from build123d import *

# Parameters (mm, degrees)
PAD_DEPTH = 10


with BuildPart() as part:
    # Sketch → Pad (new body)
    with BuildSketch(Plane.XY):
        with BuildLine():
            ThreePointArc((5, 0), (0, 5), (-5, 0))
            Line((-7, 0), (-5, 0))
            Line((-7, 7.124356), (-7, 0))
            ThreePointArc((-7, 7.124356), (-3.464466, 8.588822), (-2, 12.124356))
            Line((2, 12.124356), (-2, 12.124356))
            ThreePointArc((2, 12.124356), (3.464466, 8.588822), (7, 7.124356))
            Line((7, 0), (7, 7.124356))
            Line((5, 0), (7, 0))
        make_face()
    extrude(amount=PAD_DEPTH)


solid = part.part
The listing builds one solid part. Answer for the finished solid, in the listing's coordinates (mm). Give positions to 0.01 mm unless a question says otherwise; leave off trailing zeros. Write each loop counter-clockwise with the first axis right and the second up, starting at its lowest first coordinate (ties: lowest second). Pieces come first, ordered by that corner, then holes. Notation, with made-up numbers: (67.5, -4) - (92.5, -4) arc R15 ccw to (92.5, 13) - close; hole circle Ø2 at (41, 75.25). An arc over 180 degrees is marked (long way). One line per question, with ' | ' between items. Start each with the question number.
1. Straight lines are drawn through the part: line 1 (X direction, y = 0.5, z = 3); line 2 (X direction, y = 1.75, z = 7.25); line 3 (Y direction, x = 3, z = 3.5). For each, find the intervals that lie inside material, in ascending order.
2. Section C-C, the plane x = 0 is taken. Determine the outline of the cut face in (y, z), then the cut area to 3 significant figures.
3. Section B-B, the plane z = 8 is taken. Determine the outline of the cut face in (x, y), then the cut area to 3 significant figures.
4. Section A-A, the plane y = 4.75 is taken. Determine the outline of the cut face in (x, z).
5. Given P1, Ø5, axis at x = 1.5, z = 8.5, coming from the -Y side, flat-ended and moving along its own axis, determine where the tip first touches the part or whether it passes through.
6. Section D-D, the plane y = 9.25 is taken. Determine the outline of the cut face in (x, z), then the cut area to 3 significant figures.
Result:
1) line 1: x = -7 to -4.97, 4.97 to 7 | line 2: x = -7 to -4.68, 4.68 to 7 | line 3: y = 4 to 9.12
2) outline: (5, 0) - (12.12, 0) - (12.12, 10) - (5, 10) - close | area: 71.2 mm2
3) outline: (-7, 0) - (-5, 0) arc R5 cw to (5, 0) - (7, 0) - (7, 7.12) arc R5 cw to (2, 12.12) - (-2, 12.12) arc R5 cw to (-7, 7.12) - close | area: 91.2 mm2
4) outline: (-7, 0) - (-1.56, 0) - (-1.56, 10) - (-7, 10) - close; (1.56, 0) - (7, 0) - (7, 10) - (1.56, 10) - close
5) P1: stops at y = 3
6) outline: (-2.91, 0) - (2.91, 0) - (2.91, 10) - (-2.91, 10) - close | area: 58.2 mm2
